The model under review builds one solid part; all positions refer to its coordinate system, in mm. A direction names the side the tool comes from. Coordinates: 2 decimals unless noted, no trailing zeros. Order: outer loops, then holes, each group sorted by start corner. A loop starts at its lowest first (then second) coordinate and runs counter-clockwise, first axis right, second up. Notation, with made-up numbers: M 79,-24.5 L 121,-24.5 A17 ccw 121,8.5 Z; hole C -10,-16 d9. An arc over 180 degrees is marked long. Answer as CSV lines item,"result". Start each with the question number.
Q1. For P1, Ø2, axis at y = 3.5, z = -208.5, coming from the +X side; P2, Ø1.5, axis at x = 93.5, y = 2.5, coming from the -Z side, all flat-tipped, find the tip position at first contact; note any pin that passes through.
Q2. Consider section D-D on z = -17. Write out the cut boundary in (x, y).
Q3. Consider section C-C on x = 19. Write out the cut boundary in (y, z), and give its area (3 significant figures).
Q4. Machinability: for faces 5 (the face through (63, 2.5, -111.5)), 6 (the face through (-88.45, 2.54, -2.61)), which of the approach directions +Z, -Z, +X, -X, +Y, -Y give a long, thin tool a straight path to every point of the face, cutting with its end or side? Answer none if there is none.
Q5. The part is to be moulded in two halves that separate along Z. For faces 1 (the face through (55.85, 2.54, -122.38)), 2 (the face through (-15.591, 2.535, -66.125)), 3 (the face through (88.45, 2.54, -2.61)), 4 (the face through (-2, 0, -145)), say which applies: +Z half, -Z half, draft (parallel to the pull), parting line (faces both ways), or undercut.
Q6. Consider section A-A on x = 72. Write out the cut boundary in (y, z), and give its area (3 significant figures).
Q7. Consider section B-B on y = 3. State how many separate pieces and enclosed holes the cut face has, and give its area (3 significant figures).
Q8. Wall thickness on L1, parallel to X at y = 2.9, z = -193; L2, parallel to X at y = 2.6, z = -142; L3, parallel to Z at x = 69, y = 3.6: over which ranges is each line inside the solid? List them lowest first. Write a range as [from, to].
from build123d import *

# Parameters (mm, degrees)
EXTRUDE_1_DEPTH     = 5
FILLET_1_R          = 20
CUT_EXTRUDE_1_DEPTH = 10
FILLET_2_R          = 2


with BuildPart() as part:
    # 草圖1 → 填料-伸長1 (new body)
    with BuildSketch(Plane(origin=(0, 0, 0), x_dir=(1, 0, 0), z_dir=(0, 1, 0))):
        Polygon((-90.122176988, 0), (90.122176988, 0), (165.122176988, 129.903810568), (75, 286), (-75, 286), (-165.122176988, 129.903810568), align=None)
    extrude(amount=EXTRUDE_1_DEPTH)

    # 圓角1
    fillet_1_edges = [part.edges().sort_by_distance(p)[0] for p in [
        (-165.122176988, 2.5, -129.903810568),
        (-75, 2.5, -286),
        (75, 2.5, -286),
        (165.122176988, 2.5, -129.903810568),
        (90.122176988, 2.5, 0),
        (-90.122176988, 2.5, 0),
    ]]
    fillet(fillet_1_edges, radius=FILLET_1_R)

    # 草圖2 → 除料-伸長1 (cut)
    with BuildSketch(Plane(origin=(0, 5, 0), x_dir=(1, 0, 0), z_dir=(0, 1, 0))):
        Polygon((-11.79016319, 180.324972243), (40.171361037, 210.324972243), (33.671361037, 221.583302492), (-18.29016319, 191.583302492), align=None)
        Polygon((-44.270925304, 176.583302492), (-37.770925304, 165.324972243), (-89.732449531, 135.324972243), (-96.232449531, 146.583302492), align=None)
        Polygon((4.229074696, 92.578838325), (-47.732449531, 62.578838325), (-41.232449531, 51.320508076), (10.729074696, 81.320508076), align=None)
        Polygon((36.70983681, 96.320508076), (30.20983681, 107.578838325), (82.171361037, 137.578838325), (88.671361037, 126.320508076), align=None)
    extrude(amount=-CUT_EXTRUDE_1_DEPTH, mode=Mode.SUBTRACT)

    # 圓角2
    fillet_2_edges = [part.edges().sort_by_distance(p)[0] for p in [
        (88.671361037, 2.5, -126.320508076),
        (36.70983681, 2.5, -96.320508076),
        (30.20983681, 2.5, -107.578838325),
        (82.171361037, 2.5, -137.578838325),
        (-11.79016319, 2.5, -180.324972243),
        (-18.29016319, 2.5, -191.583302492),
        (33.671361037, 2.5, -221.583302492),
        (40.171361037, 2.5, -210.324972243),
        (-96.232449531, 2.5, -146.583302492),
        (-44.270925304, 2.5, -176.583302492),
        (-37.770925304, 2.5, -165.324972243),
        (-89.732449531, 2.5, -135.324972243),
        (4.229074696, 2.5, -92.578838325),
        (10.729074696, 2.5, -81.320508076),
        (-41.232449531, 2.5, -51.320508076),
        (-47.732449531, 2.5, -62.578838325),
    ]]
    fillet(fillet_2_edges, radius=FILLET_2_R)


solid = part.part
Evaluation:
1,P1,"stops at x = 120.32"
1,P2,"stops at z = -255.26"
2,outline,"M -99.94,0 L 99.94,0 L 99.94,5 L -99.94,5 Z"
3,outline,"M 0,-286 L 5,-286 L 5,-213.11 L 0,-213.11 Z; M 0,-198.1 L 5,-198.1 L 5,0 L 0,0 Z"
3,area,"1,350 mm²"
4,face 5,"+Y, -Y"
4,face 6,"+Z, -X, +Y, -Y"
5,face 1,"undercut"
5,face 2,"undercut"
5,face 3,"+Z half"
5,face 4,"draft"
6,outline,"M 0,-284.08 L 5,-284.08 L 5,-131.71 L 0,-131.71 Z; M 0,-116.7 L 5,-116.7 L 5,0 L 0,0 Z"
6,area,"1,350 mm²"
7,separate pieces,"1"
7,enclosed holes,"4"
7,area,"67,400 mm²"
8,L1,"x = [-128.69, -15.84], [10.16, 128.69]"
8,L2,"x = [-158.14, -93.59], [-78.17, 158.14]"
8,L3,"z = [-285.22, -129.97], [-114.96, 0]"
